Verification items for the finished model (mm, model axes). A direction names the side the tool comes from. Coordinates: 2 decimals unless noted, no trailing zeros. Write each loop counter-clockwise with the first axis right and the second up, starting at its lowest first coordinate (ties: lowest second). Pieces come first, ordered by that corner, then holes. Notation, with made-up numbers: (-15, -17) -> (28, -17) arc R18 ccw to (28, -6) -> close; hole circle Ø10 at (13, -21). An arc over 180 degrees is marked (long way). Answer in a Markdown table with one row per item.
```python
from build123d import *

# Parameters (mm, degrees)
SKETCH1_W           = 39.5
SKETCH1_H           = 43
BOSS_EXTRUDE1_DEPTH = 50


with BuildPart() as part:
    # Sketch1 → Boss-Extrude1 (new body)
    with BuildSketch(Plane.XY):
        with BuildLine():
            Line((-19.75, 48.643473355), (-19.75, 23.5))
            Line((-19.75, 23.5), (19.75, 23.5))
            Line((19.75, 23.5), (19.75, 48.643473355))
            ThreePointArc((19.75, 48.643473355), (20.754462841, 48.223461844), (21.75, 47.782711309))
            Line((21.75, 47.782711309), (21.75, 23.5))
            Line((21.75, 23.5), (46.946778377, 23.5))
            ThreePointArc((46.946778377, 23.5), (47.431791843, 22.505002168), (47.895720059, 21.5))
            Line((47.895720059, 21.5), (21.75, 21.5))
            Line((21.75, 21.5), (21.75, -21.5))
            Line((21.75, -21.5), (47.895720059, -21.5))
            ThreePointArc((47.895720059, -21.5), (47.431791843, -22.505002168), (46.946778377, -23.5))
            Line((46.946778377, -23.5), (21.75, -23.5))
            Line((21.75, -23.5), (21.75, -47.782711309))
            ThreePointArc((21.75, -47.782711309), (20.754462841, -48.223461844), (19.75, -48.643473355))
            Line((19.75, -48.643473355), (19.75, -23.5))
            Line((19.75, -23.5), (-19.75, -23.5))
            Line((-19.75, -23.5), (-19.75, -48.643473355))
            ThreePointArc((-19.75, -48.643473355), (-20.754462841, -48.223461844), (-21.75, -47.782711309))
            Line((-21.75, -47.782711309), (-21.75, -23.5))
            Line((-21.75, -23.5), (-46.946778377, -23.5))
            ThreePointArc((-46.946778377, -23.5), (-47.431791843, -22.505002168), (-47.895720059, -21.5))
            Line((-47.895720059, -21.5), (-21.75, -21.5))
            Line((-21.75, -21.5), (-21.75, 21.5))
            Line((-21.75, 21.5), (-47.895720059, 21.5))
            ThreePointArc((-47.895720059, 21.5), (-47.431791843, 22.505002168), (-46.946778377, 23.5))
            Line((-46.946778377, 23.5), (-21.75, 23.5))
            Line((-21.75, 23.5), (-21.75, 47.782711309))
            ThreePointArc((-21.75, 47.782711309), (-20.754462841, 48.223461844), (-19.75, 48.643473355))
        make_face()
        Rectangle(SKETCH1_W, SKETCH1_H, mode=Mode.SUBTRACT)
    extrude(amount=BOSS_EXTRUDE1_DEPTH)

    # Sketch2 → Cut-Revolve1 (revolve, cut)
    with BuildSketch(Plane(origin=(0, 0, 0), x_dir=(1, 0, 0), z_dir=(0, 1, 0))):
        Polygon((-52.5, -48.5), (-23.44, -64), (0, -64), (0, -76.924912946), (-62.730842365, -76.924912946), (-62.730842365, -48.5), align=None)
    revolve(axis=Axis((0, 0, -17.212629341), (0, 0, 1)), mode=Mode.SUBTRACT)


solid = part.part
```
1. Go/stop test with flat-tipped pins: pin 1 (21.5 mm diameter, centred on y = -10, z = 33.5, fed in from +X); pin 2 (10 mm diameter, centred on x = 21, z = 11, fed in from +Y); pin 3 (3 mm diameter, centred on y = -34, z = 42.5, fed in from -X). Record where each tip stops, or that it passes through.
Findings below:
| item | result |
|---|---|
| pin 1 | stops at x = 21.75 |
| pin 2 | stops at y = 48.64 |
| pin 3 | stops at x = -21.75 |
2. Material ranges on probe 1 along Y at (x, z) = (-40.5, 13.5); probe 2 along X at (y, z) = (-26.5, 42.5), recorded low to high. Write a range as from..to.
Findings below:
| item | result |
|---|---|
| probe 1 | y = -23.5..-21.5, 21.5..23.5 |
| probe 2 | x = -21.75..-19.75, 19.75..21.75 |
3. Sectioned sample at A-A, the plane y = 26. Record the cut outline in (x, z).
Findings below:
| item | result |
|---|---|
| outline | (-21.75, 0) -> (-19.75, 0) -> (-19.75, 50) -> (-21.75, 50) -> close; (19.75, 0) -> (21.75, 0) -> (21.75, 50) -> (19.75, 50) -> close |
4. Access from +Z, -Z, +X, -X, +Y, -Y to the whole of each face (thin tool, end or side, straight path). Record for faces 5 (the face through (19.75, 36, 25)), 6 (the face through (0, -21.5, 25)), 7 (the face through (-35, -21.5, 25)), 8 (the face through (-19.75, -36, 25)), 9 (the face through (-34, -23.5, 25)).
Findings below:
| item | result |
|---|---|
| face 5 | +Z, -Z, +Y |
| face 6 | +Z, -Z |
| face 7 | +Z, -Z, -X |
| face 8 | +Z, -Z, -Y |
| face 9 | +Z, -Z, -X, -Y |
5. Sectioned sample at B-B, the plane x = 18. Record the cut outline in (y, z).
Findings below:
| item | result |
|---|---|
| outline | (-23.5, 0) -> (-21.5, 0) -> (-21.5, 50) -> (-23.5, 50) -> close; (21.5, 0) -> (23.5, 0) -> (23.5, 50) -> (21.5, 50) -> close |
6. Release check for a two-part mould opening along X. For faces 1 (the face through (0, 21.5, 25)), 2 (the face through (-35, 21.5, 25)), 3 (the face through (21.75, 0, 25)), 4 (the face through (-19.75, 36, 25)) record: released by +X, released by -X, zero draft, split by the parting line, or undercut.
Findings below:
| item | result |
|---|---|
| face 1 | undercut |
| face 2 | zero draft |
| face 3 | released by +X |
| face 4 | undercut |
